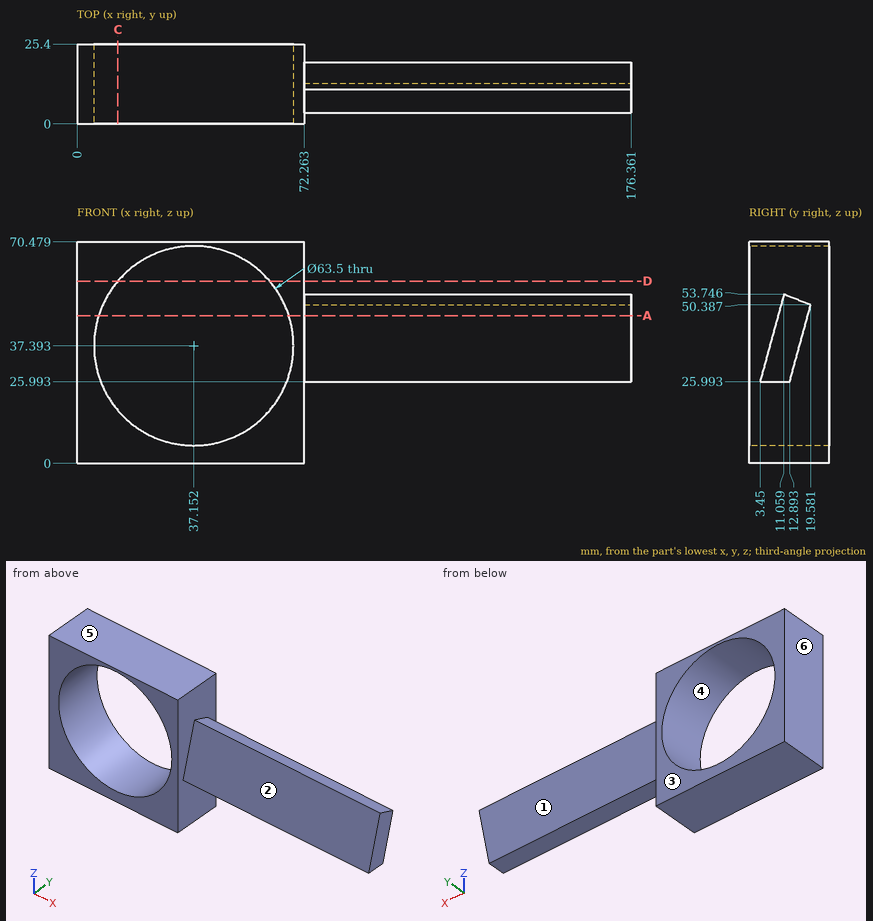
Answer from the drawing. Dimensions are ordinates in mm from the lowest x, y and z of the part. A direction names the side the tool comes from. Give positions to 0.01 mm unless a question says otherwise; leave off trailing zeros. Order: outer loops, then holes, each group sorted by start corner. A loop starts at its lowest first (then second) coordinate and runs counter-clockwise, first axis right, second up. Notation, with made-up numbers: (62, 1.25) - (118, 1.25) arc R19 ccw to (118, 26.25) - close; hole circle Ø6 at (-38, -1.5). An arc over 180 degrees is marked (long way). Use one line per item in the form item = value.
1) Consider probe 1 along Z at (x, y) = (34, 2.25) (1 decimal); probe 2 along X at (y, z) = (13.5, 13) (1 decimal); probe 3 along X at (y, z) = (12, 9.5) (1 decimal). Determine where each line is inside the solid, lowest interval first. Write a range as [from, to].
Verdict:
probe_1 = [0, 5.8], [69, 70.5]
probe_2 = [0, 16.8], [57.5, 72.3]
probe_3 = [0, 22], [52.3, 72.3]
2) Find section C-C on x = 13. Determine the outline of the cut face in (y, z), and give its area (3 significant figures).
Verdict:
outline = (0, 0) - (25.4, 0) - (25.4, 16.78) - (0, 16.78) - close; (0, 58) - (25.4, 58) - (25.4, 70.48) - (0, 70.48) - close
area = 743 mm^2
3) For the marked faces 1, 2 and 3, determine the directions among +Z, -Z, +X, -X, +Y, -Y from which every point of the face is accessible in a straight line to the end or side of a thin tool.
Verdict:
face_1 = -Z, +X, +Y
face_2 = +Z, +X, -Y
face_3 = +Z, -Z, +X, -X, +Y
4) The mould has two halves that part along X. Classify the marked faces 4, 5 and 6: released by +X, released by -X, zero draft, split by the parting line, or undercut.
Verdict:
face_4 = undercut
face_5 = zero draft
face_6 = released by -X
5) Find section A-A on z = 47. Determine the outline of the cut face in (x, y), and give its area (3 significant figures).
Verdict:
outline = (0, 0) - (6.89, 0) - (6.89, 25.4) - (0, 25.4) - close; (67.41, 0) - (72.26, 0) - (72.26, 9.21) - (176.36, 9.21) - (176.36, 18.65) - (72.26, 18.65) - (72.26, 25.4) - (67.41, 25.4) - close
area = 1,280 mm^2
6) Each of these flat-tipped pins is pushed along its axis until it touches: pin 1 (1 mm diameter, centred on y = 16, z = 17, fed in from +X); pin 2 (5 mm diameter, centred on x = 129.5, z = 38, fed in from +Y); pin 3 (1.5 mm diameter, centred on x = 86, y = 14, fed in from +Z). Where does it stop, or does it pass through?
Verdict:
pin_1 = 72.26
pin_2 = 16.87
pin_3 = 52.88
7) Find section D-D on z = 58. Determine the outline of the cut face in (x, y) (1 decimal).
Verdict:
outline = (0, 0) - (13, 0) - (13, 25.4) - (0, 25.4) - close; (61.3, 0) - (72.3, 0) - (72.3, 25.4) - (61.3, 25.4) - close
